```python
from build123d import *

# Parameters (mm, degrees)
SKETCH_1_R      = 3.5
EXTRUDE_1_DEPTH = 2


with BuildPart() as part:
    # 草图1 → 凸台-拉伸1 (new, symmetric)
    with BuildSketch(Plane.XY):
        Polygon((-115, -25), (150, -25), (150, 70), (135, 105), (-95, 105), (-115, 70), align=None)
        Circle(SKETCH_1_R, mode=Mode.SUBTRACT)
        with Locations((-80, 60)):
            Circle(SKETCH_1_R, mode=Mode.SUBTRACT)
        with Locations((120, 60)):
            Circle(SKETCH_1_R, mode=Mode.SUBTRACT)
        with Locations((-70, -5)):
            Circle(SKETCH_1_R, mode=Mode.SUBTRACT)
        with Locations((-55, 50)):
            Circle(SKETCH_1_R, mode=Mode.SUBTRACT)
        with Locations((-55, 80)):
            Circle(SKETCH_1_R, mode=Mode.SUBTRACT)
        with Locations((120, 88)):
            Circle(SKETCH_1_R, mode=Mode.SUBTRACT)
        with Locations((-80, 78)):
            Circle(SKETCH_1_R, mode=Mode.SUBTRACT)
    extrude(amount=EXTRUDE_1_DEPTH, both=True)


solid = part.part
```
Source: CAD feature listing. Evaluate the final solid. Frame: model axes, mm. Give positions to 0.01 mm unless a question says otherwise; leave off trailing zeros. Write each loop counter-clockwise with the first axis right and the second up, starting at its lowest first coordinate (ties: lowest second). Pieces come first, ordered by that corner, then holes.
1. Material intervals for line 1 along Y through (x, z) = (120, 0.7); line 2 along Y through (x, z) = (-55, 0.55); line 3 along X through (y, z) = (58, 1.6), sorted ascending.
2. Pull-direction query (X, two-part tool) for faces 1 (the face through (16, 41, 2)), 2 (the face through (-57.58, 52.365, -0.028)), 3 (the face through (-104.86, 87.745, 0.028)); classes: +X half, -X half, draft (parallel to the pull), parting line (faces both ways), or undercut.
3. Section query B-B (y = 50). Return the cut outline in (x, z), then the cut area to 3 significant figures.
4. Section query A-A (x = -80). Return the cut outline in (y, z).
5. Section query D-D (y = 88). Return the cut outline in (x, z), then the cut area to 3 significant figures.
6. Section query C-C (z = -1). Count the separate pieces of the cut face and the enclosed holes in it, then the cut area to 3 significant figures.
Output values:
1. line 1: y = -25 to 56.5, 63.5 to 84.5, 91.5 to 105
1. line 2: y = -25 to 46.5, 53.5 to 76.5, 83.5 to 105
1. line 3: x = -115 to -82.87, -77.13 to 117.13, 122.87 to 150
2. face 1: draft
2. face 2: undercut
2. face 3: -X half
3. outline: (-115, -2) - (-58.5, -2) - (-58.5, 2) - (-115, 2) - close; (-51.5, -2) - (150, -2) - (150, 2) - (-51.5, 2) - close
3. area: 1,030 mm2
4. outline: (-25, -2) - (56.5, -2) - (56.5, 2) - (-25, 2) - close; (63.5, -2) - (74.5, -2) - (74.5, 2) - (63.5, 2) - close; (81.5, -2) - (105, -2) - (105, 2) - (81.5, 2) - close
5. outline: (-104.71, -2) - (116.5, -2) - (116.5, 2) - (-104.71, 2) - close; (123.5, -2) - (142.29, -2) - (142.29, 2) - (123.5, 2) - close
5. area: 960 mm2
6. separate pieces: 1
6. enclosed holes: 8
6. area: 33,500 mm2
